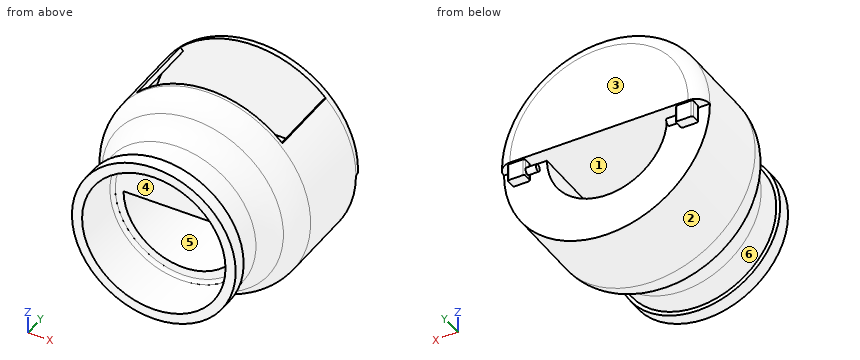
```python
from build123d import *

# Parameters (mm, degrees)
CUT_EXTRUDE3_DEPTH           = 45
CUT_EXTRUDE3_DEPTH_BACK      = 20
CUT_EXTRUDE5_START           = -5
CUT_EXTRUDE5_DEPTH           = 5
BOSS_EXTRUDE2_DEPTH          = 5
SKETCH14_R                   = 1
BOSS_EXTRUDE3_DEPTH          = 3
BOSS_EXTRUDE4_START          = 3
SKETCH15_R                   = 1
BOSS_EXTRUDE4_DEPTH          = 3
CUT_EXTRUDE6_DEPTH           = 22
SKETCH18_W                   = 1.5
SKETCH18_H                   = 21.826980301
CUT_REVOLVE1_ANGLE           = 45
CUT_REVOLVE1_OTHER_WAY_ANGLE = 45


with BuildPart() as part:
    # Sketch1 → Revolve1 (revolve)
    with BuildSketch(Plane.XY, mode=Mode.PRIVATE) as revolve1_sk:
        with BuildLine():
            Line((20.9, 0), (23.871591838, 0))
            Line((23.871591838, 0), (23.871591838, 4))
            Line((23.871591838, 4), (22.9, 4.236662843))
            Line((22.9, 4.236662843), (22.9, 11.874576818))
            ThreePointArc((22.9, 11.874576818), (23.83692213, 16.100759435), (26.472123903, 19.535021249))
            Line((26.472123903, 19.535021249), (26.427876097, 19.497892931))
            ThreePointArc((26.427876097, 19.497892931), (29.06307787, 22.932154745), (30, 27.158337362))
            Line((30, 27.158337362), (30, 50))
            ThreePointArc((30, 50), (28.828427125, 52.828427125), (26, 54))
            Line((26, 54), (0, 54))
            Line((0, 54), (0, 15))
            Line((0, 15), (19.9, 15))
            ThreePointArc((19.9, 15), (20.607106781, 14.707106781), (20.9, 14))
            Line((20.9, 14), (20.9, 0))
        make_face()
    revolve(revolve1_sk.sketch.rotate(Axis((0, 0, 0), (0, 1, 0)), 90), axis=Axis((0, 0, 0), (0, 1, 0)))

    # Sketch11 → Cut-Extrude3 (cut, two sides: drawn at the far end of the back side and taken through both)
    with BuildSketch(Plane(origin=(0, 17, 0), x_dir=(1, 0, 0), z_dir=(0, 1, 0)).offset(-CUT_EXTRUDE3_DEPTH_BACK)):
        with BuildLine():
            Line((-17.5, 0), (17.5, 0))
            ThreePointArc((17.5, 0), (0, 17.5), (-17.5, 0))
        make_face()
    extrude(amount=CUT_EXTRUDE3_DEPTH + CUT_EXTRUDE3_DEPTH_BACK, mode=Mode.SUBTRACT)

    # Sketch9 → Cut-Extrude5 (cut)
    with BuildSketch(Plane(origin=(0, 50, 0), x_dir=(-1, 0, 0), z_dir=(0, -1, 0)).offset(CUT_EXTRUDE5_START)):
        with BuildLine():
            Line((-30, 0), (30, 0))
            ThreePointArc((30, 0), (0, 30), (-30, 0))
        make_face()
    extrude(amount=CUT_EXTRUDE5_DEPTH, mode=Mode.SUBTRACT)

    # Sketch13 → Boss-Extrude2 (add)
    with BuildSketch(Plane(origin=(0, 0, 0), x_dir=(-1, 0, 0), z_dir=(0, 0, -1))):
        with BuildLine():
            Line((22.5, 53.5), (26.5, 53.5))
            ThreePointArc((26.5, 53.5), (26.853553391, 53.353553391), (27, 53))
            Line((27, 53), (27, 51))
            ThreePointArc((27, 51), (26.853553391, 50.646446609), (26.5, 50.5))
            Line((26.5, 50.5), (22.5, 50.5))
            ThreePointArc((22.5, 50.5), (22.146446609, 50.646446609), (22, 51))
            Line((22, 51), (22, 53))
            ThreePointArc((22, 53), (22.146446609, 53.353553391), (22.5, 53.5))
        make_face()
        with BuildLine():
            Line((-26.5, 53.5), (-22.5, 53.5))
            ThreePointArc((-22.5, 53.5), (-22.146446609, 53.353553391), (-22, 53))
            Line((-22, 53), (-22, 51))
            ThreePointArc((-22, 51), (-22.146446609, 50.646446609), (-22.5, 50.5))
            Line((-22.5, 50.5), (-26.5, 50.5))
            ThreePointArc((-26.5, 50.5), (-26.853553391, 50.646446609), (-27, 51))
            Line((-27, 51), (-27, 53))
            ThreePointArc((-27, 53), (-26.853553391, 53.353553391), (-26.5, 53.5))
        make_face()
    extrude(amount=BOSS_EXTRUDE2_DEPTH)

    # Sketch14 → Boss-Extrude3 (add)
    with BuildSketch(Plane.ZY.offset(-22)):
        with Locations(Location((-3, 52, 0), (0, 0, 270))):
            Circle(SKETCH14_R)
    extrude(amount=BOSS_EXTRUDE3_DEPTH)

    # Sketch15 → Boss-Extrude4 (add)
    with BuildSketch(Plane(origin=(-22, 0, 0), x_dir=(0, 0, -1), z_dir=(1, 0, 0)).offset(BOSS_EXTRUDE4_START)):
        with Locations(Location((3, 52, 0), (0, 0, 270))):
            Circle(SKETCH15_R)
    extrude(amount=-BOSS_EXTRUDE4_DEPTH)

    # Sketch16 → Cut-Extrude6 (cut)
    with BuildSketch(Plane(origin=(0, 50, 0), x_dir=(-1, 0, 0), z_dir=(0, -1, 0))):
        with BuildLine():
            Line((28.470379344, -4), (-28.470379344, -4))
            ThreePointArc((-28.470379344, -4), (0, -28.75), (28.470379344, -4))
        make_face()
    extrude(amount=CUT_EXTRUDE6_DEPTH, mode=Mode.SUBTRACT)

    # Sketch18 → Cut-Revolve1 (revolve, cut)
    with BuildSketch(Plane(origin=(0, 0, 0), x_dir=(0, 0, -1), z_dir=(1, 0, 0))):
        with Locations((-29.25, 39.08650985)):
            Rectangle(SKETCH18_W, SKETCH18_H)
    revolve(axis=Axis((0, 0, 0), (0, 1, 0)), revolution_arc=CUT_REVOLVE1_ANGLE, mode=Mode.SUBTRACT)

    # Sketch18 → Cut-Revolve1 other way (revolve, cut)
    with BuildSketch(Plane(origin=(0, 0, 0), x_dir=(0, 0, -1), z_dir=(1, 0, 0))):
        with Locations((-29.25, 39.08650985)):
            Rectangle(SKETCH18_W, SKETCH18_H)
    revolve(axis=Axis((0, 0, 0), (0, -1, 0)), revolution_arc=CUT_REVOLVE1_OTHER_WAY_ANGLE, mode=Mode.SUBTRACT)


solid = part.part
```
Model file for the job. Use its own axes, mm. Face numbers are marked on the shaded views. A direction names the side the tool comes from. Round coordinates to 2 decimals unless told otherwise and drop trailing zeros. Loops run counter-clockwise (first coordinate to the right, second up) from the corner with the lowest first, then second, coordinate; pieces in that order, holes last. Notation, with made-up numbers: M 50,68 L 87,68 A31 ccw 87,98 Z; hole C 78.25,24.25 d4. An arc over 180 degrees is marked long. Put each result on its own line as item: value. Start each with the question number.
Item 1: Cut at C-C (y = 52). List the corners of the cut face in (x, z), then the cut area to 3 significant figures.
Item 2: Mould opens along X. For the marked faces 1, 2 and 3 say: released by +X, released by -X, zero draft, split by the parting line, or undercut.
Item 3: Cut at A-A (y = 42). List the corners of the cut face in (x, z).
Item 4: Drill centre lines: line 1 along Y through (x, z) = (15.5, 5); line 2 along X through (y, z) = (6.75, 0); line 3 along X through (y, z) = (3.5, 0). Where is each one in solid material? Low to high.
Item 5: 3-axis set-ups, long thin cutter, end or side, ignore diameter. For the marked faces 4, 5 and 6: which of +Z, -Z, +X, -X, +Y, -Y reach the whole face in a straight line?
Item 6: Drop flat-ended pins along their axis: P1, Ø3, axis at x = -22, z = -21.5, coming from the +Y side; P2, Ø10, axis at x = -16, y = 25.5, coming from the -Z side; P3, Ø1, axis at y = 52.5, z = -2.5, coming from the +X side. Give the stop position or say it passes through.
Answer block:
1. outline: M -29.46,0 L -27,0 L -27,-5 L -22,-5 L -22,-4 L -19,-4 L -19,-2 L -22,-2 L -22,0 L 22,0 L 22,-2 L 19,-2 L 19,-4 L 22,-4 L 22,-5 L 27,-5 L 27,0 L 29.46,0 A29.46 ccw Z
1. area: 1,430 mm2
2. face 1: undercut
2. face 2: split by the parting line
2. face 3: zero draft
3. outline: M -28.47,4 A28.75 cw -20.33,20.33 L -21.21,21.21 A30 ccw long 21.21,21.21 L 20.33,20.33 A28.75 cw 28.47,4 Z; hole M -17.5,0 A17.5 ccw 17.5,0 Z
4. line 1: 15 to 28, 50 to 54
4. line 2: -22.9 to -20.9, 20.9 to 22.9
4. line 3: -23.87 to -20.9, 20.9 to 23.87
5. face 4: -Y
5. face 5: +Y, -Y
5. face 6: none
6. P1: y = 50
6. P2: z = -27.85
6. P3: x = 27
